```python
from build123d import *

# Parameters (mm, degrees)
F1_DEPTH = 7.62
F2_R     = 5.08
F3_R     = 2.54
F4_R     = 6.35
F5_DEPTH = 5.842
F7_DEPTH = 11.2014


with BuildPart() as f1:
    # F0 (on Top) → F1 (new body)
    with BuildSketch(Plane.XY):
        with BuildLine():
            ThreePointArc((6.35, -10.9985226281), (10.9985226281, -6.35), (12.7, 0))
            ThreePointArc((12.7, 0), (10.9985226281, 6.35), (6.35, 10.9985226281))
            Line((6.35, 10.9985226281), (6.35, -10.9985226281))
        make_face()
        with BuildLine():
            Line((6.35, -10.9985226281), (6.35, 10.9985226281))
            ThreePointArc((6.35, 10.9985226281), (0, 12.7), (-6.35, 10.9985226281))
            Line((-6.35, 10.9985226281), (-6.35, -10.9985226281))
            ThreePointArc((-6.35, -10.9985226281), (0, -12.7), (6.35, -10.9985226281))
        make_face()
        with BuildLine():
            ThreePointArc((-6.35, 10.9985226281), (0, 12.7), (6.35, 10.9985226281))
            Line((6.35, 10.9985226281), (6.35, 19.05))
            Line((6.35, 19.05), (-6.35, 19.05))
            Line((-6.35, 19.05), (-6.35, 10.9985226281))
        make_face()
        with BuildLine():
            Line((6.35, -19.05), (6.35, -10.9985226281))
            ThreePointArc((6.35, -10.9985226281), (0, -12.7), (-6.35, -10.9985226281))
            Line((-6.35, -10.9985226281), (-6.35, -19.05))
            Line((-6.35, -19.05), (6.35, -19.05))
        make_face()
        with BuildLine():
            Line((-6.35, -10.9985226281), (-6.35, 10.9985226281))
            ThreePointArc((-6.35, 10.9985226281), (-12.7, 0), (-6.35, -10.9985226281))
        make_face()
    extrude(amount=F1_DEPTH)

    # F2
    f2_edges = [f1.edges().sort_by_distance(p)[0] for p in [
        (6.35, -10.998523, 3.81),
        (6.35, -19.05, 3.81),
        (-6.35, -19.05, 3.81),
        (-6.35, -10.998523, 3.81),
        (-6.35, 10.998523, 3.81),
        (-6.35, 19.05, 3.81),
        (6.35, 19.05, 3.81),
        (6.35, 10.998523, 3.81),
    ]]
    fillet(f2_edges, radius=F2_R)

    # F3
    f3_edges = [f1.edges().sort_by_distance(p)[0] for p in [
        (12.7, 0, 7.62),
        (6.825859, -11.472541, 7.62),
        (6.825859, 11.472541, 7.62),
        (6.35, -13.794616, 7.62),
        (6.35, 13.794616, 7.62),
        (4.862102, -17.562102, 7.62),
        (4.862102, 17.562102, 7.62),
        (0, -19.05, 7.62),
        (0, 19.05, 7.62),
        (-4.862102, -17.562102, 7.62),
        (-4.862102, 17.562102, 7.62),
        (-6.35, -13.794616, 7.62),
        (-6.35, 13.794616, 7.62),
        (-6.825859, -11.472541, 7.62),
        (-6.825859, 11.472541, 7.62),
        (-12.7, 0, 7.62),
    ]]
    fillet(f3_edges, radius=F3_R)

    # F4 (on face) → F5 (join)
    with BuildSketch(Plane(origin=(0, 0, 0), x_dir=(1, 0, 0), z_dir=(0, 0, -1))):
        Circle(F4_R)
    extrude(amount=F5_DEPTH)

    # F6 (on face) → F7 (cut)
    with BuildSketch(Plane(origin=(0, 0, -5.842), x_dir=(1, 0, 0), z_dir=(0, 0, -1))):
        with BuildLine():
            Line((-2.1082, 2.3740509177), (-2.1082, -2.3740509177))
            ThreePointArc((-2.1082, -2.3740509177), (3.175, 0), (-2.1082, 2.3740509177))
        make_face()
    extrude(amount=-F7_DEPTH, mode=Mode.SUBTRACT)


solid = f1.part
```
Can you work these out from the model? Positions are in its coordinate system, mm. A direction names the side the tool comes from. Coordinates: 2 decimals unless noted, no trailing zeros. Order: outer loops, then holes, each group sorted by start corner. A loop starts at its lowest first (then second) coordinate and runs counter-clockwise, first axis right, second up.
1. If we section it at A-A (z = 1): Please give me the cut outline in (x, y) (3 decimals).
2. For faces 1 (the face through (-5.626, 13.797, 6.856)), 2 (the face through (3.173, 0.102, -0.32)), 3 (the face through (5.626, 13.792, 6.856)), which set-ups out of +Z, -Z, +X, -X, +Y, -Y let a thin tool reach every point of the face, with its end or its side?
3. I need wall thicknesses on line 1 (X direction, y = 0, z = -2.5) (3 decimals); line 2 (Y direction, x = 0, z = -1) (3 decimals); line 3 (Z direction, x = -7.25, y = 10). Which ranges of each line are inside material? Lowest first, please.
4. I'm going to push flat-ended pins straight in: pin 1 (2.5 mm diameter, centred on x = 0.5, y = 1, fed in from -Z); pin 2 (4 mm diameter, centred on y = -10, z = 3.5, fed in from +X); pin 3 (1 mm diameter, centred on y = -12.5, z = 0, fed in from +X) (3 decimals). Where does each tip first touch, or does it pass through?
5. If we section it at B-B (z = -0.75): Please give me the cut outline in (x, y) (3 decimals).
6. Thinking about a two-plate mould opening in Y: for faces 4 (the face through (0.018, 18.326, 6.856)), 5 (the face through (0, 0, 5.359)), 6 (the face through (-5.626, -13.792, 6.856)), which applies, +Y half, -Y half, draft (parallel to the pull), parting line (faces both ways), or undercut?
Entries:
1. outline: (-8.164, -9.728) arc R5.08 cw to (-6.35, -13.619) - (-6.35, -13.97) arc R5.08 ccw to (-1.27, -19.05) - (1.27, -19.05) arc R5.08 ccw to (6.35, -13.97) - (6.35, -13.619) arc R5.08 cw to (8.164, -9.728) arc R12.7 ccw to (8.164, 9.728) arc R5.08 cw to (6.35, 13.619) - (6.35, 13.97) arc R5.08 ccw to (1.27, 19.05) - (-1.27, 19.05) arc R5.08 ccw to (-6.35, 13.97) - (-6.35, 13.619) arc R5.08 cw to (-8.164, 9.728) arc R12.7 ccw to start; hole (-2.108, -2.374) arc R3.175 ccw (long way) to (-2.108, 2.374) - close
2. face 1: +Z, -X, +Y
2. face 2: -Z
2. face 3: +Z, +X, +Y
3. line 1: x = -6.35 to -2.108, 3.175 to 6.35
3. line 2: y = -6.35 to -3.175, 3.175 to 6.35
3. line 3: z = 0 to 6.52
4. pin 1: stops at z = 5.36
4. pin 2: stops at x = 9.86
4. pin 3: stops at x = 6.615
5. outline: circle Ø12.7 at (0, 0); hole (-2.108, -2.374) arc R3.175 ccw (long way) to (-2.108, 2.374) - close
6. face 4: +Y half
6. face 5: undercut
6. face 6: draft
